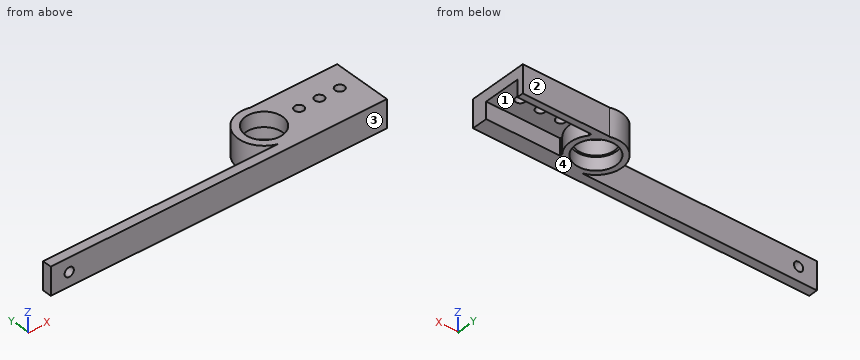
from build123d import *

# Parameters (mm, degrees)
SKETCH_1_W          = 40
SKETCH_1_H          = 20
EXTRUDE_1_DEPTH     = 6
SKETCH_2_R          = 2.5
CUT_EXTRUDE_1_DEPTH = 24.151673806
EXTRUDE_START       = -15
EXTRUDE_2_OUTLINE_R = 11
EXTRUDE_2_DEPTH     = 15
EXTRUDE_START_2     = -8
SKETCH_5_R          = 11
SKETCH_5_R_2        = 10
EXTRUDE_3_DEPTH     = 8
SKETCH_10_W         = 15
SKETCH_10_H         = 5
EXTRUDE_4_DEPTH     = 200
SKETCH_11_W         = 3.09493726
SKETCH_11_H         = 3.09493726
EXTRUDE_5_DEPTH     = 15
SKETCH_18_W         = 44.754670229
SKETCH_18_H         = 64.187168005
CUT_EXTRUDE_3_DEPTH = 184.131783151
SKETCH_19_R         = 2.5
CUT_EXTRUDE_4_DEPTH = 166.562236052


# Read off the part's stored shape, not the designer's step: 凸台-拉伸2
with BuildPart() as part:
    # 草图1 → 凸台-拉伸1 (new body)
    with BuildSketch(Plane.XY):
        Rectangle(SKETCH_1_W, SKETCH_1_H)
    extrude(amount=EXTRUDE_1_DEPTH)

    # 草图2 → 切除-拉伸1 (cut, through all)
    with BuildSketch(Plane.XY.offset(6)):
        with Locations((10, 0)):
            Circle(SKETCH_2_R)
        with Locations((-1, 0)):
            Circle(SKETCH_2_R)
        with Locations((-12, 0)):
            Circle(SKETCH_2_R)
    extrude(amount=-CUT_EXTRUDE_1_DEPTH, mode=Mode.SUBTRACT)

    # 凸台-拉伸2 outline → 凸台-拉伸2 (add)
    with BuildSketch(Plane.XY.offset(6).offset(EXTRUDE_START)):
        with BuildLine():
            Line((20, 10), (20, 13.5))
            Line((20, 13.5), (-26.893967141, 13.5))
            Line((-26.893967141, 13.5), (-26.893967141, 13.384337644))
            ThreePointArc((-26.893967141, 13.384337644), (-45, 0), (-26.893967141, -13.384337644))
            Line((-26.893967141, -13.384337644), (-26.893967141, -13.5))
            Line((-26.893967141, -13.5), (20, -13.5))
            Line((20, -13.5), (20, -10))
            Line((20, -10), (-20, -10))
            Line((-20, -10), (-20, -8.660254038))
            ThreePointArc((-20, -8.660254038), (-17, 0), (-20, 8.660254038))
            Line((-20, 8.660254038), (-20, 10))
            Line((-20, 10), (20, 10))
        make_face()
        with Locations((-31, 0)):
            Circle(EXTRUDE_2_OUTLINE_R, mode=Mode.SUBTRACT)
    extrude(amount=EXTRUDE_2_DEPTH)

    # 草图5 → 凸台-拉伸3 (add)
    with BuildSketch(Plane.XY.offset(6).offset(EXTRUDE_START_2)):
        with Locations((-31, 0)):
            Circle(SKETCH_5_R)
        with Locations((-31, 0)):
            Circle(SKETCH_5_R_2, mode=Mode.SUBTRACT)
    extrude(amount=EXTRUDE_3_DEPTH)

    # 草图10 → 凸台-拉伸4 (add)
    with BuildSketch(Plane(origin=(20, 0, 0), x_dir=(0, 0, -1), z_dir=(1, 0, 0))):
        with Locations((1.5, -16)):
            Rectangle(SKETCH_10_W, SKETCH_10_H)
    extrude(amount=-EXTRUDE_4_DEPTH)

    # 草图11 → 凸台-拉伸5 (add, through all)
    with BuildSketch(Plane.XY.offset(6)):
        with Locations((-27.071814196, -13.413570993)):
            Rectangle(SKETCH_11_W, SKETCH_11_H)
    extrude(amount=-EXTRUDE_5_DEPTH)

    # 草图18 → 切除-拉伸3 (cut, through all)
    with BuildSketch(Plane.XZ.offset(18.5)):
        with Locations((-184.468679753, -6.901085589)):
            Rectangle(SKETCH_18_W, SKETCH_18_H)
    extrude(amount=-CUT_EXTRUDE_3_DEPTH, mode=Mode.SUBTRACT)

    # 草图19 → 切除-拉伸4 (cut, through all)
    with BuildSketch(Plane.XZ.offset(18.5)):
        with Locations(Location((-152.091344638, -1.5, 0), (0, 0, 270))):
            Circle(SKETCH_19_R)
    extrude(amount=-CUT_EXTRUDE_4_DEPTH, mode=Mode.SUBTRACT)


solid = part.part
Could you check a few things on this model? Use its own coordinates, in mm. Face numbers are marked on the shaded views. Give positions to 0.01 mm unless a question says otherwise; leave off trailing zeros. Write each loop counter-clockwise with the first axis right and the second up, starting at its lowest first coordinate (ties: lowest second). Pieces come first, ordered by that corner, then holes. Notation, with made-up numbers: (81, 79.5) -> (113, 79.5) arc R16 ccw to (113, 94.5) -> close; hole circle Ø3 at (4, 65.25). An arc over 180 degrees is marked (long way). Answer as CSV lines item,"result". Start each with the question number.
(1) I'm going to push flat-ended pins straight in: pin 1 Ø4.5 at (x, z) = (7, -5.5) entering from +Y; pin 2 Ø8 at (x, z) = (-152.09, -1.5) entering from +Y; pin 3 Ø8 at (x, y) = (10, 0) entering from -Z. Where does each tip first touch, or does it pass through?
(2) Please list where these lines run through material, in increasing order: line 1 (Y direction, x = -12, z = 1.45); line 2 (Y direction, x = -31, z = -4.25); line 3 (Z direction, x = -2.5, y = -5.5).
(3) If we section it at B-B, the plane x = -12: Write out the boundary of the cut face in (y, z).
(4) If we mould it in two halves opening along Y, with no side actions, what happens to the marked faces 1, 2, 3 and 4? For each: +Y half, -Y half, draft (parallel to the pull), parting line (faces both ways), or undercut.
(5) If we section it at D-D, the plane x = -143.5: Write out the boundary of the cut face in (y, z).
(6) If we section it at A-A, the plane y = 0: Write out the boundary of the cut face in (x, z).
(7) If we section it at C-C, the plane z = -6: Write out the boundary of the cut face in (x, y), and give its area (3 significant figures).
Answer list:
1,pin 1,"y = 13.5"
1,pin 2,"y = -13.5"
1,pin 3,"z = 0"
2,line 1,"-18.5 to -2.5, 2.5 to 13.5"
2,line 2,"-18.5 to -11, 11 to 14"
2,line 3,"0 to 6"
3,outline,"(-18.5, -9) -> (-10, -9) -> (-10, 0) -> (-2.5, 0) -> (-2.5, 6) -> (-18.5, 6) -> close; (2.5, 0) -> (10, 0) -> (10, -9) -> (13.5, -9) -> (13.5, 6) -> (2.5, 6) -> close"
4,face 1,"undercut"
4,face 2,"+Y half"
4,face 3,"-Y half"
4,face 4,"draft"
5,outline,"(-18.5, -9) -> (-13.5, -9) -> (-13.5, 6) -> (-18.5, 6) -> close"
6,outline,"(-45, -9) -> (-42, -9) -> (-42, -2) -> (-41, -2) -> (-41, 6) -> (-45, 6) -> close; (-21, -2) -> (-20, -2) -> (-20, -9) -> (-17, -9) -> (-17, 0) -> (-14.5, 0) -> (-14.5, 6) -> (-21, 6) -> close; (-9.5, 0) -> (-3.5, 0) -> (-3.5, 6) -> (-9.5, 6) -> close; (1.5, 0) -> (7.5, 0) -> (7.5, 6) -> (1.5, 6) -> close; (12.5, 0) -> (20, 0) -> (20, 6) -> (12.5, 6) -> close"
7,outline,"(-162.09, -18.5) -> (20, -18.5) -> (20, -10) -> (-20, -10) -> (-20, -8.66) arc R14 ccw to (-20, 8.66) -> (-20, 10) -> (20, 10) -> (20, 13.5) -> (-26.89, 13.5) -> (-26.89, 13.38) arc R14 ccw (long way) to (-34.71, -13.5) -> (-162.09, -13.5) -> close; hole circle Ø22 at (-31, 0)"
7,area,"1,450 mm^2"
